```python
from build123d import *

# Parameters (mm, degrees)
EXTRUDE_1_DEPTH      = 1.2
CUT_EXTRUDE_START    = -1.2
CUT_EXTRUDE_1_DEPTH  = 1.2
EXTRUDE_2_DEPTH      = 0.3
EXTRUDE_2_DEPTH_BACK = 1.2
SKETCH_3_R           = 0.3
SKETCH_4_W           = 8.968131771
SKETCH_4_H           = 42.786888223
EXTRUDE_3_DEPTH      = 0.6


# Read off the part's stored shape, not the designer's step: Вырез-Вытянуть-Тонкостенный1
with BuildPart() as part:
    # Эскиз1 → Бобышка-Вытянуть1 (new body)
    with BuildSketch(Plane.XY):
        with BuildLine():
            Line((-5.411197125, -16.421197495), (2.932953168, -22.548932866))
            Line((2.932953168, -22.548932866), (7.313221262, -18.965077153))
            Line((7.313221262, -18.965077153), (5.214911567, 14.277588478))
            add(Edge.make_bspline(
                [(5.214911567, 14.277588478), (5.138438722, 15.014978004), (4.987374421, 16.471615759), (4.285048461, 18.555840063), (3.313335464, 20.541616369), (2.370787647, 21.6834935), (1.892587883, 22.262822595)],
                knots=[0, 0, 0, 0, 0.251767614, 0.497341227, 0.74497707, 1, 1, 1, 1], degree=3))
            Line((1.892587883, 22.262822595), (1.612438242, 22.548932866))
            Line((1.612438242, 22.548932866), (-7.313221262, 12.961413017))
            Line((-7.313221262, 12.961413017), (-5.451496049, -15.895327784))
            Line((-5.451496049, -15.895327784), (-5.411197125, -16.421197495))
        make_face()
    extrude(amount=EXTRUDE_1_DEPTH)

    # Вырез-Вытянуть-Тонкостенный1 outline → Вырез-Вытянуть-Тонкостенный1 (cut)
    with BuildSketch(Plane.XY.offset(1.2).offset(CUT_EXTRUDE_START)):
        with BuildLine():
            Line((7.313221262, -18.965077153), (5.214911567, 14.277588478))
            add(Edge.make_bspline(
                [(5.214911567, 14.277588478), (5.138438722, 15.014978004), (4.987374421, 16.471615759), (4.285048461, 18.555840063), (3.313335464, 20.541616369), (2.370787647, 21.6834935), (1.892587883, 22.262822595)],
                knots=[0, 0, 0, 0, 0.251767614, 0.497341227, 0.74497707, 1, 1, 1, 1], degree=3))
            Line((1.892587883, 22.262822595), (1.612438242, 22.548932866))
            Line((1.612438242, 22.548932866), (-7.313221262, 12.961413017))
            Line((-7.313221262, 12.961413017), (-5.451496049, -15.895327784))
            Line((-5.451496049, -15.895327784), (-5.411197125, -16.421197495))
            Line((-5.411197125, -16.421197495), (2.932953168, -22.548932866))
            Line((2.932953168, -22.548932866), (7.313221262, -18.965077153))
        make_face()
        with BuildLine():
            add(Edge.make_bspline(
                [(4.816213875, 14.244344904), (4.742720796, 14.952991901), (4.670057139, 15.661759974), (4.444177706, 16.707849761), (4.349214266, 17.051042697), (4.131298148, 17.722896385), (4.008075561, 18.052719847), (3.607234384, 19.028852016), (3.299546795, 19.66229506), (2.721200979, 20.562478072), (2.509851785, 20.852004475), (2.072144291, 21.416226224), (1.845069272, 21.691997878), (1.617672174, 21.967521187)],
                knots=[0, 0, 0, 0, 0.25, 0.25, 0.375, 0.375, 0.5, 0.5, 0.75, 0.75, 0.875, 0.875, 1, 1, 1, 1], degree=3))
            Line((4.816213875, 14.244344904), (6.901087174, -18.785453392))
            Line((6.901087174, -18.785453392), (2.919717459, -22.042937704))
            Line((2.919717459, -22.042937704), (-5.026399994, -16.2075077))
            Line((-5.026399994, -16.2075077), (-5.052481173, -15.867168531))
            Line((-5.052481173, -15.867168531), (-6.902948488, 12.81507484))
            Line((-6.902948488, 12.81507484), (1.617672174, 21.967521187))
        make_face(mode=Mode.SUBTRACT)
    extrude(amount=CUT_EXTRUDE_1_DEPTH, mode=Mode.SUBTRACT)

    # Эскиз3 → Бобышка-Вытянуть2 (add, two sides: drawn at the far end of the back side and taken through both)
    with BuildSketch(Plane(origin=(5.692649923, 0.359325653, 0), x_dir=(0, 0, -1), z_dir=(0.9980138039949711, 0.06299561123989302, 0)).offset(-EXTRUDE_2_DEPTH_BACK)):
        with Locations(Location((-0.6, -18.882880004, 0), (0, 0, 90))):
            Circle(SKETCH_3_R)
        with Locations(Location((-0.6, -7.882880004, 0), (0, 0, 90))):
            Circle(SKETCH_3_R)
        with Locations(Location((-0.6, 3.117119996, 0), (0, 0, 90))):
            Circle(SKETCH_3_R)
        with Locations(Location((-0.6, 14.117119996, 0), (0, 0, 90))):
            Circle(SKETCH_3_R)
    extrude(amount=EXTRUDE_2_DEPTH + EXTRUDE_2_DEPTH_BACK)

    # Эскиз4 → Бобышка-Вытянуть3 (add)
    with BuildSketch(Plane(origin=(5.992054064, 0.378224336, 0), x_dir=(0, 0, -1), z_dir=(0.9980138039949711, 0.06299561123989304, 0))):
        with Locations((-0.702688531, -0.337065509)):
            Rectangle(SKETCH_4_W, SKETCH_4_H)
    extrude(amount=EXTRUDE_3_DEPTH)


solid = part.part
```
Could you check a few things on this model? Use its own coordinates, in mm. A direction names the side the tool comes from. Round coordinates to 2 decimals unless told otherwise and drop trailing zeros. Loops run counter-clockwise (first coordinate to the right, second up) from the corner with the lowest first, then second, coordinate; pieces in that order, holes last.
Q1. I want a section at B-B (z = -1.75). Write out the boundary of the cut face in (x, y), and give its area (3 significant figures).
Q2. Please list where these lines run through material, in increasing order: L1, parallel to Z at x = -4, y = -5.5; L2, parallel to Y at x = -2, z = 1; L3, parallel to X at y = 19, z = 0.5 (3 decimals).
Q3. On a 3-axis mill with a long thin cutter (end or side, diameter ignored), from which of +Z, -Z, +X, -X, +Y, -Y can I reach the whole of each face in a straight line? I mean faces 1 (the flat face through (6.3, -0.2, 5.187)), 2 (the flat face through (4.94, -20.39, 0.59)). Say none if no direction works.
Q4. I want a section at A-A (y = -13). Write out the boundary of the cut face in (x, z).
Q5. I want a section at C-C (y = 10). Write out the boundary of the cut face in (x, z), and give its area (3 significant figures).
Q6. For P1, Ø5, axis at y = -5, z = -0.5, coming from the -X side; P2, Ø3, axis at x = -2.5, z = 3.5, coming from the -Y side; P3, Ø1, axis at y = 4.5, z = 2.5, coming from the -X side; P4, Ø8, axis at x = -2, y = -16, coming from the +Z side, each with a flat end and sliding along its axis, tell me the tip position at first contact or that it passes through.
Q7. I want a section at D-D (x = -2.25). Write out the boundary of the cut face in (y, z), and give its area (3 significant figures).
Q8. Thinking about a two-plate mould opening in Y: for faces 3 (the flat face through (5.844, -2.039, 0.592)), 4 (the flat face through (6.3, -0.2, -3.781)), 5 (the flat face through (-2.7, 17.33, 0.59)), 6 (the flat face through (-5.965, -1.727, 0.592)), which applies, pulls with the +Y half, pulls with the -Y half, needs draft (parallel to the pull), parting line crosses it, or undercut?
Answer below:
1. outline: (4.67, 21.39) - (7.36, -21.31) - (7.96, -21.27) - (5.26, 21.43) - close
1. area: 25.7 mm2
2. L1: z = 0 to 1.2
2. L2: y = -18.43 to 18.08
2. L3: x = -1.145 to 3.603, 4.817 to 5.418
3. face 1: +Z, +X, -X, +Y, -Y
3. face 2: +Z, -Z, -Y
4. outline: (-5.24, 0) - (6.54, 0) - (6.54, 1.2) - (-5.24, 1.2) - close; (6.84, -3.78) - (7.44, -3.78) - (7.44, 5.19) - (6.84, 5.19) - close
5. outline: (-6.72, 0) - (5.08, 0) - (5.08, 1.2) - (-6.72, 1.2) - close; (5.38, -3.78) - (5.99, -3.78) - (5.99, 5.19) - (5.38, 5.19) - close
5. area: 19.6 mm2
6. P1: stops at x = -5.91
6. P2: passes through
6. P3: stops at x = 5.7
6. P4: stops at z = 1.2
7. outline: (-18.25, 0) - (17.81, 0) - (17.81, 1.2) - (-18.25, 1.2) - close
7. area: 43.3 mm2
8. face 3: undercut
8. face 4: needs draft
8. face 5: pulls with the +Y half
8. face 6: pulls with the -Y half
